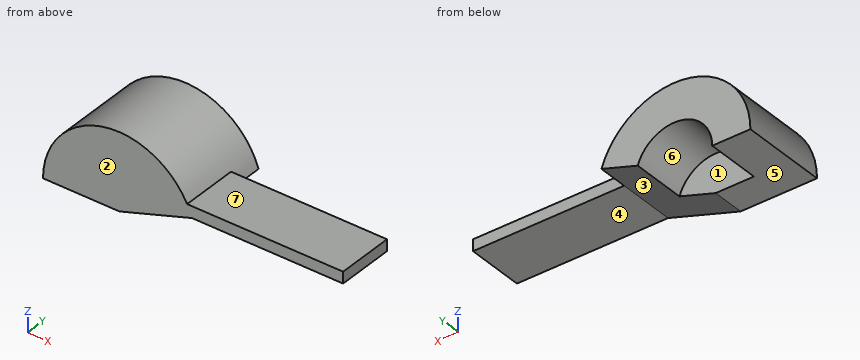
from build123d import *

# Parameters (mm, degrees)
SKETCH1_W              = 2.756398936
SKETCH1_H              = 15
REVOLVE2_ANGLE         = 180
BOSS_EXTRUDE1_START    = 6.25
SKETCH1_7_W            = 41.323169176
SKETCH1_7_H            = 15
BOSS_EXTRUDE1_DEPTH    = 3
CUT_REVOLVE2_START     = -9.499177596
CUT_REVOLVE2_OUTLINE_W = 22.75
CUT_REVOLVE2_OUTLINE_H = 7
CUT_REVOLVE2_DEPTH     = 29.499177596


with BuildPart() as part:
    # Sketch1 → Revolve2 (revolve)
    with BuildSketch(Plane.XY):
        Polygon((17.243601064, 9), (20, 9), (20, 16.75), (10, 16.75), (10, 2.5), (0, 2.5), (0, -6), (17.243601064, -6), align=None)
        with Locations((18.621800532, 1.5)):
            Rectangle(SKETCH1_W, SKETCH1_H)
    revolve(axis=Axis((0, 2.5, 0), (0, -1, 0)), revolution_arc=REVOLVE2_ANGLE)

    # Sketch1<7> → Boss-Extrude1 (add)
    with BuildSketch(Plane.XY.offset(BOSS_EXTRUDE1_START)):
        with Locations((37.905185652, 1.5)):
            Rectangle(SKETCH1_7_W, SKETCH1_7_H)
    extrude(amount=BOSS_EXTRUDE1_DEPTH)

    # Cut-Revolve2: read off the stored shape, not the designer's step
    # Cut-Revolve2 outline → Cut-Revolve2 (cut)
    with BuildSketch(Plane(origin=(0, 0, 0), x_dir=(0, 1, 0), z_dir=(0.9499177595981665, 0, 0.31250000000000017)).offset(CUT_REVOLVE2_START)):
        with Locations((5.375, -3.5)):
            Rectangle(CUT_REVOLVE2_OUTLINE_W, CUT_REVOLVE2_OUTLINE_H)
    extrude(amount=CUT_REVOLVE2_DEPTH, mode=Mode.SUBTRACT)


solid = part.part
The listing builds one solid part. Answer for the finished solid, in the listing's coordinates (mm). Face numbers are marked on the shaded views. A direction names the side the tool comes from. Round coordinates to 2 decimals unless told otherwise and drop trailing zeros. Order: outer loops, then holes, each group sorted by start corner. A loop starts at its lowest first (then second) coordinate and runs counter-clockwise, first axis right, second up. Notation, with made-up numbers: M -0.5,68 L 39.5,68 A23 cw 39.5,97 Z; hole C 64,9.5 d8. An arc over 180 degrees is marked long. Answer in a Markdown table with one row per item. Add a question column.
1) The part is cut by section C-C on x = -8. Determine the outline of the cut face in (y, z).
2) The part is cut by section B-B on y = -0.25. Determine the outline of the cut face in (x, z), plus the area to 3 significant figures.
3) The part is cut by section A-A on z = 7.75. Determine the outline of the cut face in (x, y), plus the area to 3 significant figures.
4) Determine the mould class of the marked faces 1, 2 and 3 for opening direction X: pulls with the +X half, pulls with the -X half, needs draft (parallel to the pull), parting line crosses it, or undercut.
5) Consider line 1 along Z through (x, y) = (53, 4.5); line 2 along Y through (x, z) = (2, 7.5); line 3 along X through (y, z) = (13.5, 15.25). Determine where each line is inside the solid, lowest interval first. Write a range as from..to.
6) Which of the six approach directions +Z, -Z, +X, -X, +Y, -Y give full straight-line access (tool end or side, diameter ignored) to the marked faces 4, 5, 6 and 7?
7) Flat-ended cylindrical pins translate along their axes: pin 1 Ø3 at (x, y) = (16.5, 1.5) entering from +Z; pin 2 Ø10 at (x, y) = (11.5, 5) entering from +Z; pin 3 Ø12 at (x, y) = (31.5, 4) entering from +Z. Find the tip coordinate at first contact, or state that the pin passes through.
8) The part is cut by section D-D on x = 24.5. Determine the outline of the cut face in (y, z).
Findings below:
| question | item | result |
|---|---|---|
| 1 | outline | M -6,0 L 2.5,0 L 2.5,6 L 16.75,6 L 16.75,18.33 L -6,18.33 Z |
| 2 | outline | M -20,0 L 0,0 L 19,6.25 L 58.57,6.25 L 58.57,9.25 L 17.73,9.25 A20 ccw Z |
| 2 | area | 685 mm² |
| 3 | outline | M -18.44,-6 L 58.57,-6 L 58.57,9 L 18.44,9 L 18.44,16.75 L 6.32,16.75 L 6.32,2.5 L -6.32,2.5 L -6.32,16.75 L -18.44,16.75 Z |
| 3 | area | 1,260 mm² |
| 4 | face 1 | undercut |
| 4 | face 2 | needs draft |
| 4 | face 3 | pulls with the +X half |
| 5 | line 1 | z = 6.25..9.25 |
| 5 | line 2 | y = -6..2.5 |
| 5 | line 3 | x = -12.94..12.94 |
| 6 | face 4 | -Z, +X, +Y, -Y |
| 6 | face 5 | -Z, +X, -X, +Y, -Y |
| 6 | face 6 | -Z, +Y |
| 6 | face 7 | +Z, +X, +Y, -Y |
| 7 | pin 1 | stops at z = 13.23 |
| 7 | pin 2 | stops at z = 18.91 |
| 7 | pin 3 | stops at z = 9.25 |
| 8 | outline | M -6,6.25 L 9,6.25 L 9,9.25 L -6,9.25 Z |
